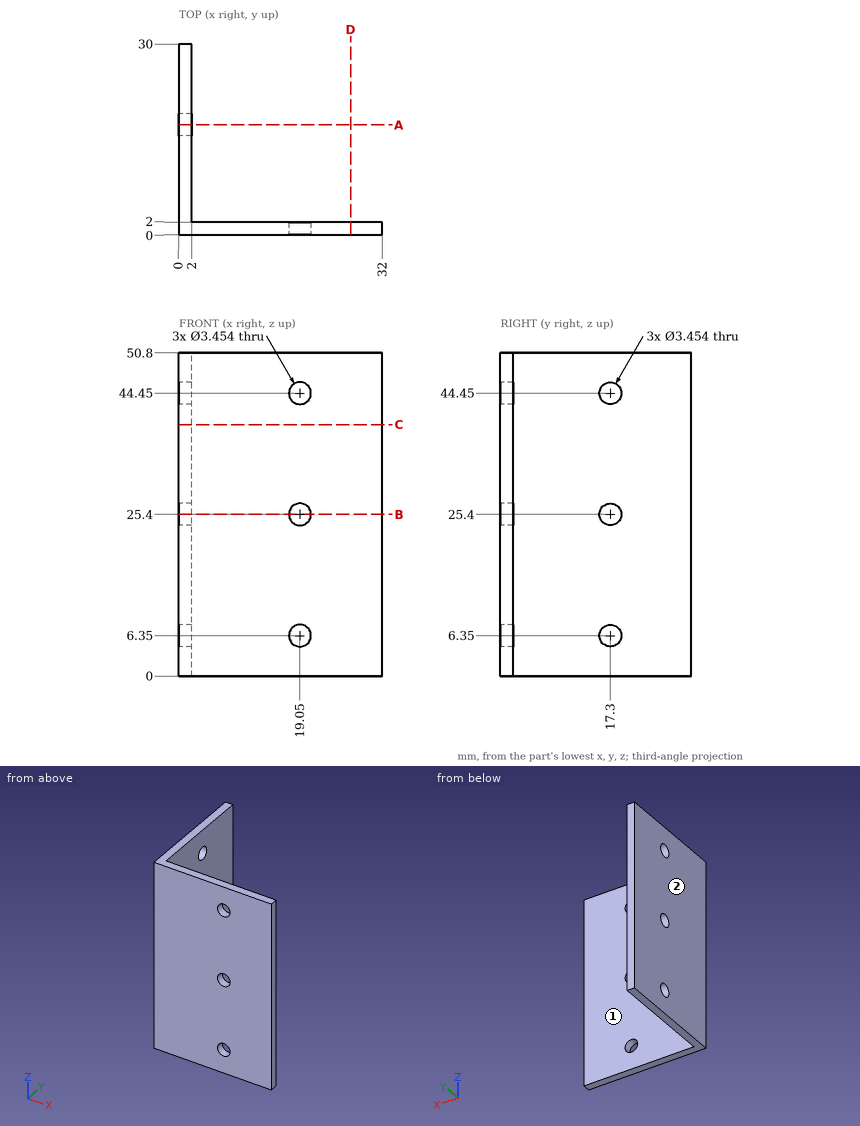
Check sheet for the drawn part. Datum: minimum x, y, z corner. Units: mm. A direction names the side the tool comes from. Round coordinates to 2 decimals unless told otherwise and drop trailing zeros. Order: outer loops, then holes, each group sorted by start corner. A loop starts at its lowest first (then second) coordinate and runs counter-clockwise, first axis right, second up. Notation, with made-up numbers: M 50.25,81 L 54.25,81 A18 ccw 54.25,96 Z; hole C 45.5,60 d11. An arc over 180 degrees is marked long. Answer in a Markdown table with one row per item.
(1) Gauge pin test, flat ends, axial feed: pin 1 (5.5 mm diameter, centred on y = 17.3, z = 6.35, fed in from +X); pin 2 (3 mm diameter, centred on x = 19.05, z = 6.35, fed in from -Y); pin 3 (3 mm diameter, centred on x = 4, z = 9, fed in from +Y). Record the tip position at first contact, or that the pin passes through.
Findings:
| item | result |
|---|---|
| pin 1 | stops at x = 2 |
| pin 2 | passes through |
| pin 3 | stops at y = 2 |
(2) Section check B-B on z = 25.4. Record the boundary of the cut face in (x, y), plus the area to 3 significant figures.
Findings:
| item | result |
|---|---|
| outline | M 0,0 L 17.32,0 L 17.32,2 L 2,2 L 2,15.57 L 0,15.57 Z; M 0,19.03 L 2,19.03 L 2,30 L 0,30 Z; M 20.78,0 L 32,0 L 32,2 L 20.78,2 Z |
| area | 106 mm^2 |
(3) Material ranges on line 1 along Z through (x, y) = (19.05, 1.4); line 2 along Y through (x, z) = (1.65, 25.4); line 3 along X through (y, z) = (1.55, 6.35), recorded low to high. Write a range as from..to.
Findings:
| item | result |
|---|---|
| line 1 | z = 0..4.62, 8.08..23.67, 27.13..42.72, 46.18..50.8 |
| line 2 | y = 0..15.57, 19.03..30 |
| line 3 | x = 0..17.32, 20.78..32 |
(4) Set-up check for the marked faces 1 and 2: record each of +Z, -Z, +X, -X, +Y, -Y from which the full face is reachable in a straight line by a thin tool's end or side.
Findings:
| item | result |
|---|---|
| face 1 | +Z, -Z, +X, +Y |
| face 2 | +Z, -Z, -X, +Y, -Y |
(5) Section check D-D on x = 27. Record the boundary of the cut face in (y, z), plus the area to 3 significant figures.
Findings:
| item | result |
|---|---|
| outline | M 0,0 L 2,0 L 2,50.8 L 0,50.8 Z |
| area | 102 mm^2 |
(6) Section check A-A on y = 17.3. Record the boundary of the cut face in (x, z).
Findings:
| item | result |
|---|---|
| outline | M 0,0 L 2,0 L 2,4.62 L 0,4.62 Z; M 0,8.08 L 2,8.08 L 2,23.67 L 0,23.67 Z; M 0,27.13 L 2,27.13 L 2,42.72 L 0,42.72 Z; M 0,46.18 L 2,46.18 L 2,50.8 L 0,50.8 Z |
(7) Section check C-C on z = 39.5. Record the boundary of the cut face in (x, y).
Findings:
| item | result |
|---|---|
| outline | M 0,0 L 32,0 L 32,2 L 2,2 L 2,30 L 0,30 Z |
